Autodesk Inventor part; units mm, degrees
ref_plane "YZ Plane" through (0, 0, 0) normal (1, 0, 0) x (0, 1, 0)
ref_plane "XZ Plane" through (0, 0, 0) normal (0, 1, 0) x (-1, 0, 0)
ref_plane "XY Plane" through (0, 0, 0) normal (0, 0, 1) x (1, 0, 0)
sketch "Эскиз1" plane through (0, 0, 0) normal (0, 0, 1) x (1, 0, 0)
  circle A0 centre (0, 0) radius 12.5
  circle A1 centre (0, 0) radius 26
  line L0 (0, -26) -> (-70, -26)
  line L1 (-70, -26) -> (70, -26)
  line L2 (70, -26) -> (70, -11)
  line L3 (70, -11) -> (-70, -11)
  line L4 (-70, -11) -> (-70, -26)
  line L5 (0, -26) -> (-15, -26)
  line L6 (-15, -26) -> (-15, -23)
  line L7 (-15, -23) -> (15, -23)
  line L8 (15, -23) -> (15, -26)
  point P0 (23.5584, -11)
  point P1 (-23.5584, -11)
  dimension "d1" = 52
  dimension "d0" = 25
  dimension "d2" = 70
  dimension "d5" = 15
  dimension "d6" = 15
  dimension "d7" = 3
  dimension "d8" = 30
extrude "Выдавливание1" add sketch "Эскиз1" along normal blind 38 contours A0 L3 A1 | A0 L3 A1 L7 | A1 L7 L6 L0 L4 L3 | L3 L2 L1 L8 L7 A1
sketch "Эскиз2" plane through (-70, -11, 0) normal (0, 1, 0) x (1, 0, 0)
  line L0 (0, 0) -> (0, -38)
  line L1 (85, 0) -> (140, 0)
  line L2 (0, -38) -> (140, -38)
  line L3 (140, -38) -> (140, 0)
  line L4 (140, 0) -> (0, 0)
  line L5 (0, 0) -> (0, -38)
  line L6 (70, 0) -> (70, -38)
  line L7 (70, -19) -> (122.5, -19)
  line L8 (122.5, -19) -> (17.5, -19)
  line L9 (17.5, -19) -> (19, -19)
  line L10 (19, -19) -> (16, -19)
  arc A0 (16, -12.5) -> (16, -25.5) centre (16, -19) ccw
  arc A1 (19, -25.5) -> (19, -12.5) centre (19, -19) ccw
  line L11 (16, -25.5) -> (19, -25.5)
  line L12 (19, -12.5) -> (16, -12.5)
  line L13 (122.5, -19) -> (121, -19)
  line L14 (121, -19) -> (124, -19)
  arc A2 (124, -25.5) -> (124, -12.5) centre (124, -19) ccw
  arc A3 (121, -12.5) -> (121, -25.5) centre (121, -19) ccw
  line L15 (121, -25.5) -> (124, -25.5)
  line L16 (121, -12.5) -> (124, -12.5)
  dimension "d11" = 52.5
  dimension "d12" = 105
  dimension "d13" = 1.5
  dimension "d14" = 3
  dimension "d15" = 13
  dimension "d16" = 1.5
  dimension "d17" = 3
extrude "Выдавливание2" cut sketch "Эскиз2" against normal blind 53.75 contours A1 L11 A0 L12 | A3 L16 A2 L15
properties part number "Подшипник качения 25 мм ГОСТ 8338-75"
The model under review builds one solid part; all positions refer to its coordinate system, in mm. A direction names the side the tool comes from. Round coordinates to 2 decimals unless told otherwise and drop trailing zeros. Loops run counter-clockwise (first coordinate to the right, second up) from the corner with the lowest first, then second, coordinate; pieces in that order, holes last. Notation, with made-up numbers: M 77.25,-26 L 105.25,-26 A10 ccw 105.25,-22 Z; hole C 55,10.5 d10. An arc over 180 degrees is marked long. Write item = value, one per line.
Item 1: For line 1 (Y direction, x = 0, z = 8); line 2 (X direction, y = 0, z = 10); line 3 (Y direction, x = -34.5, z = 26), list the stretches that pass through material, from the lowest coordinate up. Write a range as [from, to].
Return value:
line_1 = [-23, -12.5], [12.5, 26]
line_2 = [-26, -12.5], [12.5, 26]
line_3 = [-26, -11]
Item 2: The part is to be moulded in two halves that separate along Z. For faces 4 (the flat face through (-1, -17, 38)), 5 (the flat face through (-53, -18, 25.5)), 6 (the flat face through (15, -24, 19)), say which applies: released by +Z, released by -Z, zero draft, split by the parting line, or undercut.
Return value:
face_4 = released by +Z
face_5 = undercut
face_6 = zero draft
Item 3: Take a section at D-D on z = 31.5. Write out the cut boundary in (x, y).
Return value:
outline = M -70,-26 L -15,-26 L -15,-23 L 15,-23 L 15,-26 L 70,-26 L 70,-11 L 23.56,-11 A26 ccw long -23.56,-11 L -70,-11 Z; hole C 0,0 d25
Item 4: Take a section at A-A on z = 19. Write out the cut boundary in (x, y).
Return value:
outline = M -70,-26 L -60.5,-26 L -60.5,-11 L -70,-11 Z; M -44.5,-26 L -15,-26 L -15,-23 L 15,-23 L 15,-26 L 44.5,-26 L 44.5,-11 L 23.56,-11 A26 ccw long -23.56,-11 L -44.5,-11 Z; M 60.5,-26 L 70,-26 L 70,-11 L 60.5,-11 Z; hole C 0,0 d25
Item 5: Take a section at B-B on y = 10. Write out the cut boundary in (x, z), then the cut area to 3 significant figures.
Return value:
outline = M -24,0 L -7.5,0 L -7.5,38 L -24,38 Z; M 7.5,0 L 24,0 L 24,38 L 7.5,38 Z
area = 1,250 mm2
Item 6: Insertion check: P1, Ø6, axis at x = 8.5, z = 33, coming from the +Y side; P2, Ø11.5, axis at x = -55, z = 17, coming from the +Y side; P3, Ø1, axis at x = -7, z = 31.5, coming from the +Y side. Each pin has a flat end and moves straight along its axis. Give the tip position at first contact, or say it passes through.
Return value:
P1 = 25.41
P2 = -11
P3 = 25.17
Item 7: Take a section at C-C on x = 0. Write out the cut boundary in (y, z), then the cut area to 3 significant figures.
Return value:
outline = M -23,0 L -12.5,0 L -12.5,38 L -23,38 Z; M 12.5,0 L 26,0 L 26,38 L 12.5,38 Z
area = 912 mm2
Item 8: Machinability: for faces 1 (the flat face through (-52, -18, 12.5)), 2 (the flat face through (0, -23, 19)), 3 (the flat face through (-1, -17, 0)), which of the approach directions +Z, -Z, +X, -X, +Y, -Y give a long, thin tool a straight path to every point of the face, cutting with its end or side? Answer none if there is none.
Return value:
face_1 = +Y, -Y
face_2 = +Z, -Z, -Y
face_3 = -Z, +X, -X, +Y, -Y
